```python
from build123d import *
from OCP.BRepFilletAPI import BRepFilletAPI_MakeChamfer

# Parameters (mm, degrees)
BOSS_EXTRUDE1_DEPTH       = 17.5
FILLET1_R                 = 1
CHAMFER1_SIZE             = 4
CHAMFER1_SIZE2            = 1.07179677
F_4_CLEARANCE_HOLE1_D     = 2.9464
F_4_CLEARANCE_HOLE1_DEPTH = 6.35
CUT_EXTRUDE3_START        = -2.286
CUT_EXTRUDE3_DEPTH        = 29.572
SKETCH8_W                 = 8.65
SKETCH8_H                 = 11
CUT_EXTRUDE2_DEPTH        = 10
F_4_CLEARANCE_HOLE2_D     = 2.9464


with BuildPart() as part:
    # Sketch1 → Boss-Extrude1 (new body)
    with BuildSketch(Plane.XY):
        Polygon((-47.5, 6.35), (-35.5, 6.35), (-35.5, 31.35), (-47.5, 31.35), (-47.5, 43.85), (-35.5, 43.85), (-35.5, 37.5), (35.5, 37.5), (35.5, 0), (29.5, 0), (29.5, 30.5), (23.5, 30.5), (23.5, 31.5), (11.5, 31.5), (11.5, 30.5), (5.5, 30.5), (5.5, 0), (-5.5, 0), (-5.5, 30.5), (-11.5, 30.5), (-11.5, 31.5), (-23.5, 31.5), (-23.5, 30.5), (-29.5, 30.5), (-29.5, 0), (-47.5, 0), align=None)
    extrude(amount=BOSS_EXTRUDE1_DEPTH)

    # Fillet1
    fillet1_edges = [part.edges().sort_by_distance(p)[0] for p in [
        (-11.5, 30.5, 8.75),
        (-23.5, 30.5, 8.75),
        (23.5, 30.5, 8.75),
        (11.5, 30.5, 8.75),
    ]]
    fillet(fillet1_edges, radius=FILLET1_R - 0.0001)  # a hair under: the kernel refuses the full size

    # Chamfer1: one chamfer whose edges measure the first distance from different faces: ONE call of the kernel's chamfer builder (chamfer() names one face for all edges)
    chamfer1_edges_1 = [part.edges().sort_by_distance(p)[0] for p in [
        (5.5, 0, 8.75),
    ]]
    chamfer1_side_1 = [part.faces().sort_by_distance(p)[0] for p in [
        (5.5, 15.25, 8.75),
    ]]
    chamfer1_edges_2 = [part.edges().sort_by_distance(p)[0] for p in [
        (-5.5, 0, 8.75),
    ]]
    chamfer1_side_2 = [part.faces().sort_by_distance(p)[0] for p in [
        (-5.5, 15.25, 8.75),
    ]]
    chamfer1 = BRepFilletAPI_MakeChamfer(part.part.solid().wrapped)
    for e in chamfer1_edges_1:
        chamfer1.Add(CHAMFER1_SIZE, CHAMFER1_SIZE2, e.wrapped, chamfer1_side_1[0].wrapped)  # the first distance lies on this face
    for e in chamfer1_edges_2:
        chamfer1.Add(CHAMFER1_SIZE, CHAMFER1_SIZE2, e.wrapped, chamfer1_side_2[0].wrapped)  # the first distance lies on this face
    add(Compound.cast(chamfer1.Shape()), mode=Mode.REPLACE)

    # #4 Clearance Hole1
    with Locations(Plane(origin=(0, 6.35, 0), x_dir=(1, 0, 0), z_dir=(0, 1, 0))):
        with Locations((-41.5, -4.5), (-41.5, -13)):
            Hole(F_4_CLEARANCE_HOLE1_D / 2, depth=F_4_CLEARANCE_HOLE1_DEPTH)

    # Sketch9 → Cut-Extrude3 (cut)
    with BuildSketch(Plane(origin=(0, 6.35, 0), x_dir=(1, 0, 0), z_dir=(0, 1, 0)).offset(CUT_EXTRUDE3_START)):
        Polygon((-41.5, -9.333825791), (-44.675, -11.166912895), (-44.675, -14.833087105), (-41.5, -16.666174209), (-38.325, -14.833087105), (-38.325, -11.166912895), align=None)
        Polygon((-38.325, -6.333087105), (-38.325, -2.666912895), (-41.5, -0.833825791), (-44.675, -2.666912895), (-44.675, -6.333087105), (-41.5, -8.166174209), align=None)
    extrude(amount=CUT_EXTRUDE3_DEPTH, mode=Mode.SUBTRACT)

    # Sketch8 → Cut-Extrude2 (cut)
    with BuildSketch(Plane.ZY.offset(35.5)):
        with Locations((10.175, 17.5)):
            Rectangle(SKETCH8_W, SKETCH8_H)
    extrude(amount=-CUT_EXTRUDE2_DEPTH, mode=Mode.SUBTRACT)

    # #4 Clearance Hole2 (through all)
    with Locations(Plane(origin=(0, 31.35, 0), x_dir=(-1, 0, 0), z_dir=(0, -1, 0))):
        with Locations((41.5, -13), (41.5, -4.5)):
            Hole(F_4_CLEARANCE_HOLE2_D / 2)

    # Mirror1: part across plane


with BuildPart() as part_1:
    add(part.part)
    add(part.part.mirror(Plane(origin=(35.5, 37.5, 17.5), x_dir=(0, 0, 1), z_dir=(-1, 0, 0))))


solid = part_1.part
```
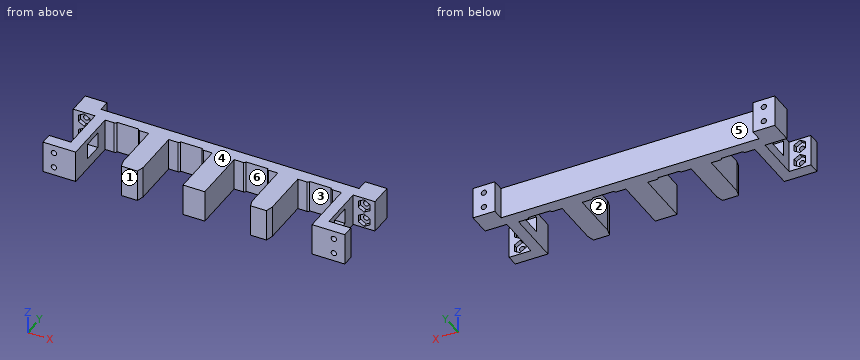
Work out the finished part from the listing and answer in its coordinate system (mm). Face numbers are marked on the shaded views. A direction names the side the tool comes from. Give positions to 0.01 mm unless a question says otherwise; leave off trailing zeros. Order: outer loops, then holes, each group sorted by start corner. A loop starts at its lowest first (then second) coordinate and runs counter-clockwise, first axis right, second up.
1. Section A-A, the plane y = 25.5 is taken. Determine the outline of the cut face in (x, z), and give its area (3 significant figures).
Result sheet:
outline: (-35.5, 0) - (-29.5, 0) - (-29.5, 17.5) - (-35.5, 17.5) - close; (-5.5, 0) - (5.5, 0) - (5.5, 17.5) - (-5.5, 17.5) - close; (29.5, 0) - (41.5, 0) - (41.5, 17.5) - (29.5, 17.5) - close; (65.5, 0) - (76.5, 0) - (76.5, 17.5) - (65.5, 17.5) - close; (100.5, 0) - (106.5, 0) - (106.5, 17.5) - (100.5, 17.5) - close
area: 805 mm2
2. Straight lines are drawn through the part: L1, parallel to Z at x = -41.5, y = 37.75; L2, parallel to X at y = 25, z = 2.5; L3, parallel to X at y = 36.75, z = 13. For each, find the intervals that lie inside material, in ascending order.
Result sheet:
L1: z = 0 to 3.03, 5.97 to 11.53, 14.47 to 17.5
L2: x = -35.5 to -29.5, -5.5 to 5.5, 29.5 to 41.5, 65.5 to 76.5, 100.5 to 106.5
L3: x = -47.5 to -42.97, -40.03 to 111.03, 113.97 to 118.5
3. For the marked faces 4, 5 and 6, determine the directions among +Z, -Z, +X, -X, +Y, -Y from which every point of the face is accessible in a straight line to the end or side of a thin tool.
Result sheet:
face 4: +Z, +X, -X, +Y, -Y
face 5: +Z, -Z, +Y
face 6: +Z, -Z, -Y
4. The mould has two halves that part along X. Classify the marked faces 1, 2 and 3: released by +X, released by -X, zero draft, split by the parting line, or undercut.
Result sheet:
face 1: zero draft
face 2: undercut
face 3: undercut
5. Section B-B, the plane x = 98 is taken. Determine the outline of the cut face in (y, z), and give its area (4 significant figures).
Result sheet:
outline: (30.5, 0) - (37.5, 0) - (37.5, 17.5) - (30.5, 17.5) - close
area: 122.5 mm2
6. Each of these flat-tipped pins is pushed along its axis until it touches: P1, Ø2, axis at y = 24, z = 14, coming from the -X side; P2, Ø4, axis at x = 80, z = 8, coming from the -Y side; P3, Ø8, axis at y = 10, z = 10, coming from the -X side; P4, Ø1, axis at x = 73, y = 38.5, coming from the +Z side. Where does it stop, or does it pass through?
Result sheet:
P1: stops at x = -35.5
P2: stops at y = 30.5
P3: stops at x = -47.5
P4: passes through
